The figure shows three views and two pictorial views of one solid part (mm, origin at its lowest corner). Answer the questions. A direction names the side the tool comes from. Coordinates: 2 decimals unless noted, no trailing zeros. Write each loop counter-clockwise with the first axis right and the second up, starting at its lowest first coordinate (ties: lowest second). Pieces come first, ordered by that corner, then holes.
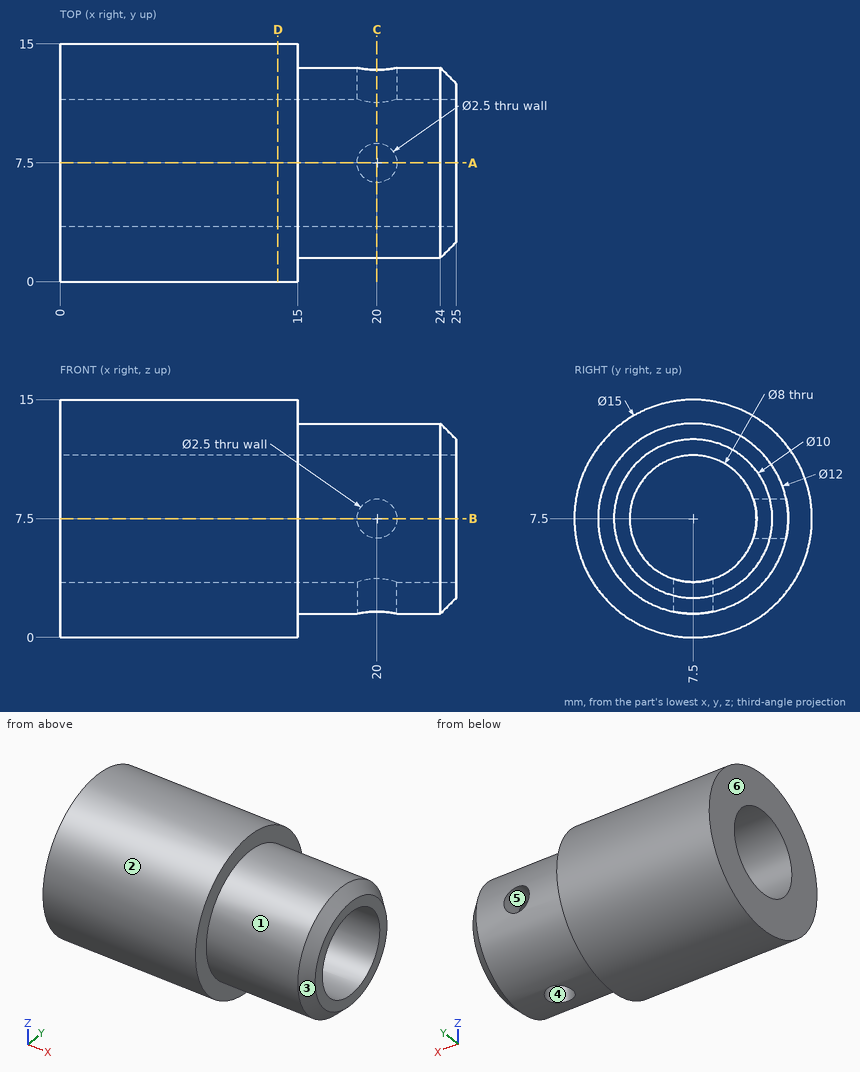
1. Section A-A on y = 7.5 is taken. Give the vertices of the cut face in (x, z).
Results found:
outline: (0, 0) - (15, 0) - (15, 1.5) - (18.75, 1.5) - (18.75, 3.5) - (0, 3.5) - close; (0, 11.5) - (25, 11.5) - (25, 12.5) - (24, 13.5) - (15, 13.5) - (15, 15) - (0, 15) - close; (21.25, 1.5) - (24, 1.5) - (25, 2.5) - (25, 3.5) - (21.25, 3.5) - close
2. Section B-B on z = 7.5 is taken. Give the vertices of the cut face in (x, y).
Results found:
outline: (0, 0) - (15, 0) - (15, 1.5) - (24, 1.5) - (25, 2.5) - (25, 3.5) - (0, 3.5) - close; (0, 11.5) - (18.75, 11.5) - (18.75, 13.5) - (15, 13.5) - (15, 15) - (0, 15) - close; (21.25, 11.5) - (25, 11.5) - (25, 12.5) - (24, 13.5) - (21.25, 13.5) - close
3. Section C-C on x = 20 is taken. Give the vertices of the cut face in (y, z).
Results found:
outline: (6.25, 1.63) - (6.25, 3.7) arc R4 cw (long way) to (11.3, 8.75) - (13.37, 8.75) arc R6 ccw (long way) to start; (8.75, 1.63) arc R6 ccw to (13.37, 6.25) - (11.3, 6.25) arc R4 cw to (8.75, 3.7) - close
4. Section D-D on x = 13.75 is taken. Give the vertices of the cut face in (y, z).
Results found:
outline: circle Ø15 at (7.5, 7.5); hole circle Ø8 at (7.5, 7.5)
5. Flat-ended cylindrical pins translate along their axes: P1, Ø2, axis at x = 21.5, z = 4.5, coming from the -Y side; P2, Ø2, axis at y = 4, z = 6.5, coming from the +X side; P3, Ø1, axis at x = 7, y = 2, coming from the -Z side; P4, Ø3, axis at x = 20, y = 7.5, coming from the -Z side. Find the tip coordinate at first contact, or state that the pin passes through.
Results found:
P1: stops at y = 1.84
P2: stops at x = 25
P3: stops at z = 1.91
P4: stops at z = 1.5
6. For a pull along X with two mould halves and no side action, classify the marked faces 3, 4, 5 and 6 as pulls with the +X half, pulls with the -X half, needs draft (parallel to the pull), parting line crosses it, or undercut.
Results found:
face 3: pulls with the +X half
face 4: undercut
face 5: undercut
face 6: pulls with the -X half
7. A tool of negligible diameter and unlimited length cuts with its end or side. For the marked faces 1 and 2, from which of +Z, -Z, +X, -X, +Y, -Y can it reach the whole face along a straight path? Write none if from no direction.
Results found:
face 1: +X
face 2: +X, -X
8. Find the intervals of material crossed by L1, parallel to Y at x = 12, z = 7.5; L2, parallel to X at y = 7.5, z = 2.9; L3, parallel to X at y = 3.25, z = 12.25, in increasing order.
Results found:
L1: y = 0 to 3.5, 11.5 to 15
L2: x = 0 to 18.75, 21.25 to 25
L3: x = 0 to 15
